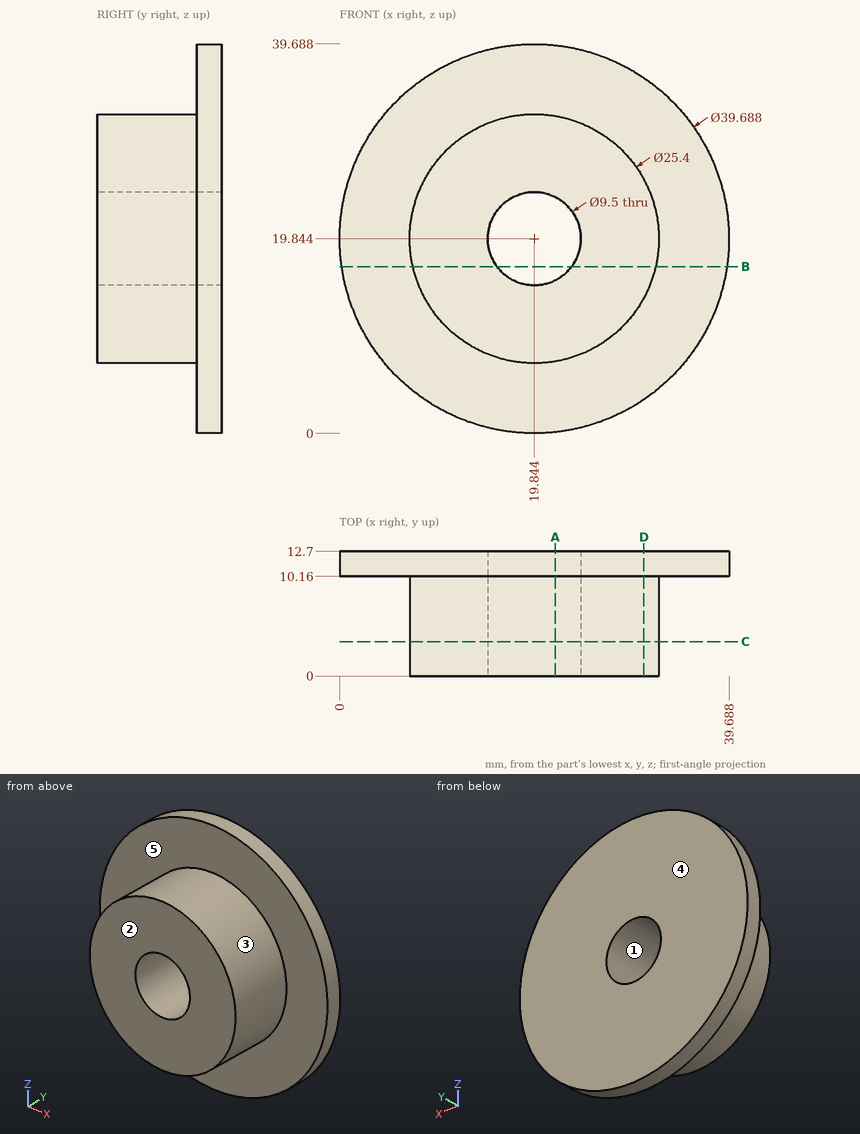
Geometry check sheet. Reference: drawing and pictorial views, mm from the part's lowest x, y, z. A direction names the side the tool comes from. Give positions to 0.01 mm unless a question says otherwise; leave off trailing zeros. Loops run counter-clockwise (first coordinate to the right, second up) from the corner with the lowest first, then second, coordinate; pieces in that order, holes last. Notation, with made-up numbers: (-29, 47.5) -> (28, 47.5) arc R27 cw to (28, 70.5) -> close; hole circle Ø1 at (31, 33.25). An arc over 180 degrees is marked (long way). Answer in a Markdown table with one row per item. Add a question column.
1) Cross-section at D-D on x = 31. Record the boundary of the cut face in (y, z) (1 decimal).
2) Set-up check for the marked faces 4 and 5: record each of +Z, -Z, +X, -X, +Y, -Y from which the full face is reachable in a straight line by a thin tool's end or side.
3) Cross-section at C-C on y = 3.5. Record the boundary of the cut face in (x, z).
4) Cross-section at A-A on x = 22. Record the boundary of the cut face in (y, z) (1 decimal), and give its area (3 significant figures).
5) Gauge pin test, flat ends, axial feed: P1, Ø1.5, axis at y = 5, z = 28, coming from the +X side; P2, Ø1, axis at x = 33.5, y = 2.5, coming from the -Z side; P3, Ø5, axis at x = 17.5, y = 3, coming from the -Z side; P4, Ø6, axis at y = 3, z = 12.5, coming from the +X side. Record the tip position at first contact, or that the pin passes through.
6) Draft check along Z on the marked faces 1, 2 and 3. Enter one of: pulls with the +Z half, pulls with the -Z half, needs draft (parallel to the pull), parting line crosses it, or undercut.
7) Material ranges on probe 1 along X at (y, z) = (3.75, 20) (1 decimal); probe 2 along Y at (x, z) = (11, 29.5); probe 3 along X at (y, z) = (3.75, 16.5) (1 decimal), recorded low to high. Write a range as from..to.
8) Cross-section at B-B on z = 17. Record the boundary of the cut face in (x, y) (1 decimal).
Outcome:
| question | item | result |
|---|---|---|
| 1 | outline | (0, 13.8) -> (10.2, 13.8) -> (10.2, 3.4) -> (12.7, 3.4) -> (12.7, 36.3) -> (10.2, 36.3) -> (10.2, 25.9) -> (0, 25.9) -> close |
| 2 | face 4 | +Z, -Z, +X, -X, +Y |
| 2 | face 5 | -Y |
| 3 | outline | circle Ø25.4 at (19.84, 19.84); hole circle Ø9.5 at (19.84, 19.84) |
| 4 | outline | (0, 7.3) -> (10.2, 7.3) -> (10.2, 0.1) -> (12.7, 0.1) -> (12.7, 15.6) -> (0, 15.6) -> close; (0, 24.1) -> (12.7, 24.1) -> (12.7, 39.6) -> (10.2, 39.6) -> (10.2, 32.4) -> (0, 32.4) -> close |
| 4 | area | 247 mm^2 |
| 5 | P1 | stops at x = 30.16 |
| 5 | P2 | passes through |
| 5 | P3 | stops at z = 7.14 |
| 5 | P4 | stops at x = 31.78 |
| 6 | face 1 | undercut |
| 6 | face 2 | needs draft |
| 6 | face 3 | parting line crosses it |
| 7 | probe 1 | x = 7.1..15.1, 24.6..32.5 |
| 7 | probe 2 | y = 10.16..12.7 |
| 7 | probe 3 | x = 7.6..16.5, 23.2..32.1 |
| 8 | outline | (0.2, 10.2) -> (7.5, 10.2) -> (7.5, 0) -> (16, 0) -> (16, 12.7) -> (0.2, 12.7) -> close; (23.6, 0) -> (32.2, 0) -> (32.2, 10.2) -> (39.5, 10.2) -> (39.5, 12.7) -> (23.6, 12.7) -> close |
